from build123d import *

# Parameters (mm, degrees)
SKETCH1_R           = 10
BOSS_EXTRUDE1_DEPTH = 11
SKETCH3_W           = 41
SKETCH3_H           = 10
BOSS_EXTRUDE2_DEPTH = 37
SKETCH4_R           = 10
CUT_EXTRUDE1_DEPTH  = 37
BOSS_EXTRUDE3_START = -11
SKETCH5_W           = 41
SKETCH5_H           = 37
SKETCH5_R           = 10
BOSS_EXTRUDE3_DEPTH = 11


with BuildPart() as part:
    # Sketch1 → Boss-Extrude1 (new body)
    with BuildSketch(Plane(origin=(0, 0, 0), x_dir=(1, 0, 0), z_dir=(0, 1, 0))):
        with BuildLine():
            Line((0, 0), (-46, 0))
            Line((-46, 0), (-46, 24))
            Line((-46, 24), (-84, 0))
            Line((-84, 0), (-125, 0))
            Line((-125, 0), (-125, 56))
            Line((-125, 56), (-22, 56))
            ThreePointArc((-22, 56), (-6.443650814, 49.556349186), (0, 34))
            Line((0, 34), (0, 0))
        make_face()
        with Locations(Location((-22, 34, 0), (0, 0, 270))):
            Circle(SKETCH1_R, mode=Mode.SUBTRACT)
    extrude(amount=BOSS_EXTRUDE1_DEPTH)

    # Sketch3 → Boss-Extrude2 (add)
    with BuildSketch(Plane(origin=(0, 11, 0), x_dir=(1, 0, 0), z_dir=(0, 1, 0))):
        with Locations((-104.5, 5)):
            Rectangle(SKETCH3_W, SKETCH3_H)
    extrude(amount=BOSS_EXTRUDE2_DEPTH)

    # Sketch4 → Cut-Extrude1 (cut)
    with BuildSketch(Plane.XY):
        with Locations((-104.5, 27)):
            Circle(SKETCH4_R)
    extrude(amount=-CUT_EXTRUDE1_DEPTH, mode=Mode.SUBTRACT)

    # Sketch5 → Boss-Extrude3 (add)
    with BuildSketch(Plane(origin=(0, 0, -56), x_dir=(-1, 0, 0), z_dir=(0, 0, -1)).offset(BOSS_EXTRUDE3_START)):
        with Locations((104.5, 29.5)):
            Rectangle(SKETCH5_W, SKETCH5_H)
        with Locations(Location((104.5, 27, 0), (0, 0, 180))):
            Circle(SKETCH5_R, mode=Mode.SUBTRACT)
    extrude(amount=BOSS_EXTRUDE3_DEPTH)


solid = part.part
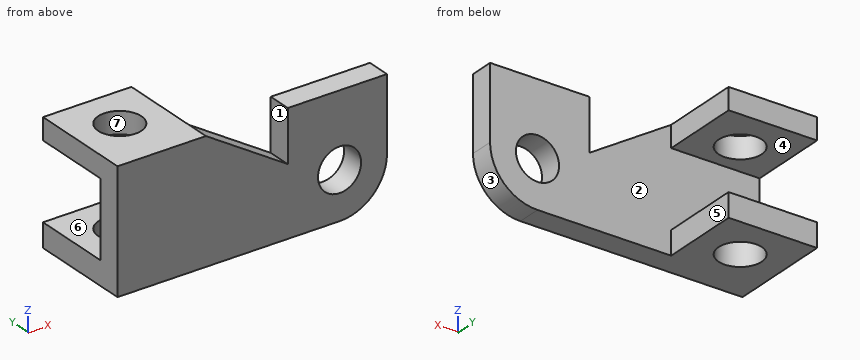
The model under review builds one solid part; all positions refer to its coordinate system, in mm. Face numbers are marked on the shaded views. A direction names the side the tool comes from. Give positions to 0.01 mm unless a question says otherwise; leave off trailing zeros. Loops run counter-clockwise (first coordinate to the right, second up) from the corner with the lowest first, then second, coordinate; pieces in that order, holes last. Notation, with made-up numbers: (71, -22) -> (124, -22) arc R18 cw to (124, -2) -> close; hole circle Ø4 at (18.25, 46.25). An arc over 180 degrees is marked (long way). Answer as a JSON object with one key per item and string values. Group by question number.
Q1. Insertion check: pin 1 (17 mm diameter, centred on x = -52.5, z = -37.5, fed in from +Y); pin 2 (10 mm diameter, centred on y = 33.5, z = -44, fed in from +X); pin 3 (18 mm diameter, centred on x = -104.5, y = 27, fed in from -Z); pin 4 (3 mm diameter, centred on x = -65, y = 8, fed in from +Z). Each pin has a flat end and moves straight along its axis. Give the tip position at first contact, or say it passes through.
Q2. Draft analysis for pull direction Z (two halves, no side actions). For the marked faces 1, 2, 3 and 4, state which applies: pulls with the +Z half, pulls with the -Z half, needs draft (parallel to the pull), parting line crosses it, or undercut.
Q3. Take a section at D-D (y = 13.5). Write out the cut boundary in (x, z), plus the area to 3 significant figures.
Q4. Take a section at A-A (y = 7). Write out the cut boundary in (x, z).
Q5. Tool access review of the marked faces 5, 6 and 7: name each direction out of +Z, -Z, +X, -X, +Y, -Y from which nothing blocks a thin tool from reaching the whole face with its end or side.
Q6. Take a section at B-B (x = -104.5). Write out the cut boundary in (y, z), plus the area to 3 significant figures.
Q7. Take a section at C-C (y = 27). Write out the cut boundary in (x, z), plus the area to 3 significant figures.
Q8. Wall thickness on line 1 along X through (y, z) = (27, -53.25); line 2 along Y through (x, z) = (-104.5, -52); line 3 along Z through (x, y) = (-97, 40.5): over which ranges is each line inside the solid? List them lowest first.
Answer below:
{
 "1": {"pin 1": "stops at y = 11", "pin 2": "stops at x = -84", "pin 3": "passes through", "pin 4": "stops at z = -11.05"},
 "2": {"face 1": "needs draft", "face 2": "undercut", "face 3": "pulls with the -Z half", "face 4": "undercut"},
 "3": {"outline": "(-125, -56) -> (-84, -56) -> (-84, -45) -> (-125, -45) -> close; (-125, -10) -> (-84, -10) -> (-84, 0) -> (-125, 0) -> close", "area": "861 mm2"},
 "4": {"outline": "(-125, -56) -> (-22, -56) arc R22 ccw to (0, -34) -> (0, 0) -> (-46, 0) -> (-46, -24) -> (-84, 0) -> (-125, 0) -> close; hole circle Ø20 at (-22, -34)"},
 "5": {"face 5": "+Z, -Z, +X, +Y", "face 6": "+X, -X, +Y", "face 7": "+Z, -Z"},
 "6": {"outline": "(0, -56) -> (17, -56) -> (17, -45) -> (11, -45) -> (11, -10) -> (17, -10) -> (17, 0) -> (0, 0) -> close; (37, -56) -> (48, -56) -> (48, -45) -> (37, -45) -> close; (37, -10) -> (48, -10) -> (48, 0) -> (37, 0) -> close", "area": "973 mm2"},
 "7": {"outline": "(-125, -56) -> (-114.5, -56) -> (-114.5, -45) -> (-125, -45) -> close; (-125, -10) -> (-114.5, -10) -> (-114.5, 0) -> (-125, 0) -> close; (-94.5, -56) -> (-84, -56) -> (-84, -45) -> (-94.5, -45) -> close; (-94.5, -10) -> (-84, -10) -> (-84, 0) -> (-94.5, 0) -> close", "area": "441 mm2"},
 "8": {"line 1": "x = -125 to -114.5, -94.5 to -84", "line 2": "y = 0 to 17, 37 to 48", "line 3": "z = -56 to -45, -10 to 0"}
}
